from build123d import *

# Parameters (mm, degrees)
SKETCH_1_R          = 1
EXTRUDE_1_DEPTH     = 2
EXTRUDE_2_DEPTH     = 4
CUT_EXTRUDE_1_DEPTH = 1


with BuildPart() as part:
    # 草圖1 → 填料-伸長1 (new body)
    with BuildSketch(Plane(origin=(0, 0, 0), x_dir=(1, 0, 0), z_dir=(0, 1, 0))):
        with BuildLine():
            Line((0, -2), (0, 2))
            Line((0, 2), (6, 2))
            ThreePointArc((6, 2), (6.707106781, 1.707106781), (7, 1))
            Line((7, 1), (7, 0))
            Line((7, 0), (7, -1))
            ThreePointArc((7, -1), (6.707106781, -1.707106781), (6, -2))
            Line((6, -2), (0, -2))
        make_face()
        with Locations((5, 0)):
            Circle(SKETCH_1_R, mode=Mode.SUBTRACT)
    extrude(amount=EXTRUDE_1_DEPTH)

    # 草圖4 → 填料-伸長2 (add)
    with BuildSketch(Plane(origin=(0, 0, 0), x_dir=(1, 0, 0), z_dir=(0, 1, 0))):
        Polygon((0, 0), (0, 2), (3, 2), (3, 1), (1, 1), (1, -1), (3, -1), (3, -2), (0, -2), align=None)
    extrude(amount=EXTRUDE_2_DEPTH)

    # 草圖5 → 除料-伸長1 (cut)
    with BuildSketch(Plane.XY.offset(2)):
        Polygon((3, 2), (1, 4), (3, 4), align=None)
    extrude(amount=-CUT_EXTRUDE_1_DEPTH, mode=Mode.SUBTRACT)


solid = part.part
Can you work these out from the model? Positions are in its coordinate system, mm. A direction names the side the tool comes from. Give positions to 0.01 mm unless a question says otherwise; leave off trailing zeros. Loops run counter-clockwise (first coordinate to the right, second up) from the corner with the lowest first, then second, coordinate; pieces in that order, holes last. Notation, with made-up numbers: (26, -32.5) - (76, -32.5) arc R33 ccw to (76, -0.5) - close; hole circle Ø1 at (-6.5, 76.25). An arc over 180 degrees is marked (long way). Return JSON: item names as keys, results as strings.
1. We'd pull the mould along Z, two halves only. Please class faces 4 (the face through (3, 2, 0)), 5 (the face through (2, 3, -1)), 6 (the face through (3, 3, -1.5)), 7 (the face through (6.699, 0.986, -1.715)): +Z half, -Z half, draft (parallel to the pull), parting line (faces both ways), or undercut.
Output values:
{"face 4": "undercut", "face 5": "undercut", "face 6": "draft", "face 7": "-Z half"}
2. I want a section at A-A on x = 5. Please give me the cut outline in (y, z), and give its area (3 significant figures).
Output values:
{"outline": "(0, -2) - (2, -2) - (2, -1) - (0, -1) - close; (0, 1) - (2, 1) - (2, 2) - (0, 2) - close", "area": "4.00 mm²"}
3. I'm going to push flat-ended pins straight in: pin 1 Ø1.2 at (x, z) = (5, 0) entering from +Y; pin 2 Ø2 at (x, z) = (5.5, -0.5) entering from +Y; pin 3 Ø1.6 at (y, z) = (3.5, 0.5) entering from +X; pin 4 Ø1 at (y, z) = (3, 1.5) entering from -X. Where does each tip first touch, or does it pass through?
Output values:
{"pin 1": "passes through", "pin 2": "stops at y = 2", "pin 3": "stops at x = 2.12", "pin 4": "stops at x = 0"}
4. If I drill on line 1 (X direction, y = 0.8, z = 0); line 2 (Z direction, x = 1.5, y = 2.5); line 3 (Y direction, x = 3.5, z = 0.15), over which ranges is the centre line in solid material (lowest first)?
Output values:
{"line 1": "x = 0 to 4, 6 to 7", "line 2": "z = -2 to -1, 1 to 2", "line 3": "y = 0 to 2"}
5. I want a section at B-B on z = 0. Please give me the cut outline in (x, y).
Output values:
{"outline": "(0, 0) - (4, 0) - (4, 2) - (1, 2) - (1, 4) - (0, 4) - close; (6, 0) - (7, 0) - (7, 2) - (6, 2) - close"}
6. I want a section at D-D on x = 2. Please give me the cut outline in (y, z), and give its area (3 significant figures).
Output values:
{"outline": "(0, -2) - (4, -2) - (4, -1) - (2, -1) - (2, 1) - (3, 1) - (3, 2) - (0, 2) - close", "area": "11.0 mm²"}
7. For faces 1 (the face through (1, 3, 0)), 2 (the face through (2, 2, 2)), 3 (the face through (2, 3, 1.5)), which set-ups out of +Z, -Z, +X, -X, +Y, -Y let a thin tool reach every point of the face, with its end or its side?
Output values:
{"face 1": "+X, +Y", "face 2": "+Z, +X, -X, +Y, -Y", "face 3": "+Z, +X, +Y"}
8. I want a section at C-C on y = 2.9. Please give me the cut outline in (x, z), and give its area (3 significant figures).
Output values:
{"outline": "(0, -2) - (3, -2) - (3, -1) - (1, -1) - (1, 1) - (2.1, 1) - (2.1, 2) - (0, 2) - close", "area": "7.10 mm²"}
